from build123d import *

# Parameters (mm, degrees)
SKETCH1_W           = 24.13
SKETCH1_H           = 25.4
SKETCH1_R           = 9.145310151
BOSS_EXTRUDE1_DEPTH = 2.54
SKETCH4_R           = 8.765161433
BOSS_EXTRUDE2_DEPTH = 7.62
BOSS_EXTRUDE3_START = -2.54
BOSS_EXTRUDE3_DEPTH = 5.08


with BuildPart() as part:
    # Sketch1 → Boss-Extrude1 (new body)
    with BuildSketch(Plane(origin=(0, 0, 0), x_dir=(1, 0, 0), z_dir=(0, 1, 0))):
        with Locations((-18.379392523, -7.539883178)):
            Rectangle(SKETCH1_W, SKETCH1_H)
        with Locations((-18.379392523, -7.539883178)):
            Circle(SKETCH1_R, mode=Mode.SUBTRACT)
        with Locations((5.750607477, -7.539883178)):
            Rectangle(SKETCH1_W, SKETCH1_H)
        with Locations((5.750607477, -7.539883178)):
            Circle(SKETCH1_R, mode=Mode.SUBTRACT)
        with Locations((5.750607477, -7.539883178)):
            Circle(SKETCH1_R)
        with Locations((-18.379392523, -7.539883178)):
            Circle(SKETCH1_R)
    extrude(amount=BOSS_EXTRUDE1_DEPTH)

    # Sketch4 → Boss-Extrude2 (add)
    with BuildSketch(Plane(origin=(0, 2.54, 0), x_dir=(1, 0, 0), z_dir=(0, 1, 0))):
        with Locations(Location((5.750607477, -7.539883178, 0), (0, 0, 90))):
            Circle(SKETCH4_R)
        with Locations(Location((-18.379392523, -7.539883178, 0), (0, 0, 90))):
            Circle(SKETCH4_R)
    extrude(amount=BOSS_EXTRUDE2_DEPTH)

    # Sketch5 → Boss-Extrude3 (add)
    with BuildSketch(Plane(origin=(0, 2.54, 0), x_dir=(1, 0, 0), z_dir=(0, 1, 0)).offset(BOSS_EXTRUDE3_START)):
        with BuildLine():
            Line((-9.642774863, 3.459380336), (-2.569962391, 3.459380336))
            ThreePointArc((-2.569962391, 3.459380336), (-1.217807066, 2.10722501), (-2.569962391, 0.755069685))
            Line((-2.569962391, 0.755069685), (-9.642774863, 0.755069685))
            ThreePointArc((-9.642774863, 0.755069685), (-10.994930189, 2.10722501), (-9.642774863, 3.459380336))
        make_face()
    extrude(amount=BOSS_EXTRUDE3_DEPTH)


solid = part.part
Verification items for the finished model (mm, model axes). A direction names the side the tool comes from. Coordinates: 2 decimals unless noted, no trailing zeros. Write each loop counter-clockwise with the first axis right and the second up, starting at its lowest first coordinate (ties: lowest second). Pieces come first, ordered by that corner, then holes. Notation, with made-up numbers: (-21.75, -25.5) - (-4.75, -25.5) arc R12 ccw to (-4.75, -4.5) - close; hole circle Ø10 at (8, -39.5). An arc over 180 degrees is marked (long way). Answer as a JSON object with one key per item and string values.
(1) Thickness scan on line 1 along Y through (x, z) = (-27, 13.75); line 2 along Z through (x, y) = (6, 9); line 3 along X through (y, z) = (5, 15.5). Record the ranges inside material, lowest first.
Report:
{"line 1": "0 to 2.54", "line 2": "-1.22 to 16.3", "line 3": "-22.05 to -14.71, 2.08 to 9.42"}
(2) Cross-section at D-D on y = 3.5. Record the cut outline in (x, z).
Report:
{"outline": "circle Ø17.53 at (-18.38, 7.54); (-9.64, -3.46) - (-2.57, -3.46) arc R1.35 ccw to (-2.57, -0.76) - (-9.64, -0.76) arc R1.35 ccw to start; circle Ø17.53 at (5.75, 7.54)"}
(3) Gauge pin test, flat ends, axial feed: pin 1 Ø3 at (x, z) = (-7, -2.5) entering from +Y; pin 2 Ø1.3 at (x, y) = (-6.5, 4.5) entering from +Z. Record the tip position at first contact, or that the pin passes through.
Report:
{"pin 1": "y = 5.08", "pin 2": "z = -0.76"}
(4) Tool access check on faces 4 (the flat face through (-19, 10.16, 8)), 5 (the flat face through (-6, 5.08, -2)), 6 (the flat face through (-7, 2.54, 7)). Record the directions out of +Z, -Z, +X, -X, +Y, -Y that give a thin tool (end or side, any length) a straight path to the whole face; none if there is none.
Report:
{"face 4": "+Z, -Z, +X, -X, +Y", "face 5": "-Z, +Y", "face 6": "+Y"}
(5) Cross-section at B-B on y = 9.5. Record the cut outline in (x, z).
Report:
{"outline": "circle Ø17.53 at (-18.38, 7.54); circle Ø17.53 at (5.75, 7.54)"}
(6) Mould release check, pull along Z, two halves, no side actions. Record for faces 1 (the flat face through (-6, 4, -3.459)), 2 (the flat face through (-30.444, 1, 8)), 3 (the cylindrical face through (-10.995, 3.792, -2.077)): pulls with the +Z half, pulls with the -Z half, needs draft (parallel to the pull), parting line crosses it, or undercut.
Report:
{"face 1": "pulls with the -Z half", "face 2": "needs draft", "face 3": "undercut"}
(7) Cross-section at A-A on x = -7. Record the cut outline in (y, z), plus the area to 3 significant figures.
Report:
{"outline": "(0, -5.16) - (2.54, -5.16) - (2.54, -3.46) - (5.08, -3.46) - (5.08, -0.76) - (2.54, -0.76) - (2.54, 20.24) - (0, 20.24) - close", "area": "71.4 mm^2"}
(8) Cross-section at C-C on z = 11. Record the cut outline in (x, y).
Report:
{"outline": "(-30.44, 0) - (17.82, 0) - (17.82, 2.54) - (13.8, 2.54) - (13.8, 10.16) - (-2.3, 10.16) - (-2.3, 2.54) - (-10.33, 2.54) - (-10.33, 10.16) - (-26.43, 10.16) - (-26.43, 2.54) - (-30.44, 2.54) - close"}
